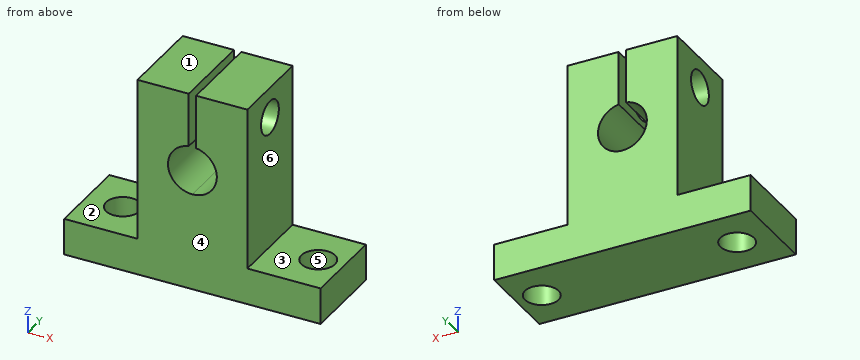
```python
from build123d import *

# Parameters (mm, degrees)
F1_DEPTH = 14
F2_R     = 2.75
F3_DEPTH = 6
F4_R     = 2.75
F5_DEPTH = 9
F6_R     = 2.75
F7_DEPTH = 9


with BuildPart() as f1:
    # F0 (on Front) → F1 (new body)
    with BuildSketch(Plane.XZ):
        with BuildLine():
            Line((-66.492734, 17.676073), (-45.492734, 17.676073))
            Line((-45.492734, 17.676073), (-24.492734, 17.676073))
            Line((-24.492734, 17.676073), (-24.492734, 23.676073))
            Line((-24.492734, 23.676073), (-36.492734, 23.676073))
            Line((-36.492734, 23.676073), (-36.492734, 50.476073))
            Line((-36.492734, 50.476073), (-44.892734, 50.476073))
            Line((-44.892734, 50.476073), (-44.892734, 41.630817))
            ThreePointArc((-44.892734, 41.630817), (-41.504064, 37.375221), (-45.492734, 33.676073))
            ThreePointArc((-45.492734, 33.676073), (-49.481404, 37.375221), (-46.092734, 41.630817))
            Line((-46.092734, 41.630817), (-46.092734, 50.476073))
            Line((-46.092734, 50.476073), (-54.492734, 50.476073))
            Line((-54.492734, 50.476073), (-54.492734, 23.676073))
            Line((-54.492734, 23.676073), (-66.492734, 23.676073))
            Line((-66.492734, 23.676073), (-66.492734, 17.676073))
        make_face()
    extrude(amount=F1_DEPTH)

    # F2 (on face) → F3 (cut)
    with BuildSketch(Plane.XY.offset(23.676073)):
        with Locations((-60.588689, -6.999696)):
            Circle(F2_R)
        with Locations((-28.588689, -6.999696)):
            Circle(F2_R)
    extrude(amount=-F3_DEPTH, mode=Mode.SUBTRACT)

    # F4 (on face) → F5 (cut)
    with BuildSketch(Plane.YZ.offset(-36.492734)):
        with Locations((-7, 45.476073)):
            Circle(F4_R)
    extrude(amount=-F5_DEPTH, mode=Mode.SUBTRACT)

    # F6 (on face) → F7 (cut)
    with BuildSketch(Plane(origin=(-54.492734, 0, 0), x_dir=(0, -1, 0), z_dir=(-1, 0, 0))):
        with Locations((7, 45.476073)):
            Circle(F6_R)
    extrude(amount=-F7_DEPTH, mode=Mode.SUBTRACT)


solid = f1.part
```
The listing builds one solid part. Answer for the finished solid, in the listing's coordinates (mm). Face numbers are marked on the shaded views. A direction names the side the tool comes from. Give positions to 0.01 mm unless a question says otherwise; leave off trailing zeros. Order: outer loops, then holes, each group sorted by start corner. A loop starts at its lowest first (then second) coordinate and runs counter-clockwise, first axis right, second up. Notation, with made-up numbers: (27.5, 66) - (74.5, 66) arc R24 cw to (74.5, 90) - close; hole circle Ø7 at (-9.75, -38.75). An arc over 180 degrees is marked (long way). Answer in a Markdown table with one row per item. Add a question column.
Q1. For a pull along Y with two mould halves and no side action, classify the marked faces 4, 5 and 6 as released by +Y, released by -Y, zero draft, split by the parting line, or undercut.
Q2. The part is cut by section D-D (y = -7.5). Determine the outline of the cut face in (x, z), then the cut area to 3 significant figures.
Q3. Find the intervals of material crossed by line 1 along X through (y, z) = (-13, 48); line 2 along X through (y, z) = (-9, 37.5); line 3 along Z through (x, y) = (-51.5, -7), in increasing order. Write a range as [from, to].
Q4. Given P1, Ø2.5, axis at y = -4.5, z = 46.5, coming from the -X side; P2, Ø6, axis at x = -31.5, y = -10.5, coming from the +Z side; P3, Ø1.5, axis at y = -6, z = 37.5, coming from the +X side, each flat-ended and moving along its own axis, determine where each tip first touches the part or whether it passes through.
Q5. The part is cut by section A-A (z = 36.5). Determine the outline of the cut face in (x, y).
Q6. The part is cut by section B-B (y = -2.5). Determine the outline of the cut face in (x, z), then the cut area to 3 significant figures.
Q7. Which of the six approach directions +Z, -Z, +X, -X, +Y, -Y give full straight-line access (tool end or side, diameter ignored) to the marked faces 1, 2 and 3?
Q8. The part is cut by section C-C (x = -59). Determine the outline of the cut face in (y, z).
Determined:
| question | item | result |
|---|---|---|
| 1 | face 4 | released by -Y |
| 1 | face 5 | undercut |
| 1 | face 6 | zero draft |
| 2 | outline | (-66.49, 17.68) - (-63.29, 17.68) - (-63.29, 23.68) - (-66.49, 23.68) - close; (-57.88, 17.68) - (-31.29, 17.68) - (-31.29, 23.68) - (-36.49, 23.68) - (-36.49, 42.77) - (-44.89, 42.77) - (-44.89, 41.63) arc R4 cw (long way) to (-46.09, 41.63) - (-46.09, 42.77) - (-54.49, 42.77) - (-54.49, 23.68) - (-57.88, 23.68) - close; (-54.49, 48.18) - (-46.09, 48.18) - (-46.09, 50.48) - (-54.49, 50.48) - close; (-44.89, 48.18) - (-36.49, 48.18) - (-36.49, 50.48) - (-44.89, 50.48) - close; (-25.88, 17.68) - (-24.49, 17.68) - (-24.49, 23.68) - (-25.88, 23.68) - close |
| 2 | area | 518 mm² |
| 3 | line 1 | x = [-54.49, -46.09], [-44.89, -36.49] |
| 3 | line 2 | x = [-54.49, -49.49], [-41.5, -36.49] |
| 3 | line 3 | z = [17.68, 42.73], [48.23, 50.48] |
| 4 | P1 | stops at x = -54.49 |
| 4 | P2 | stops at z = 23.68 |
| 4 | P3 | stops at x = -36.49 |
| 5 | outline | (-54.49, -14) - (-49.32, -14) - (-49.32, 0) - (-54.49, 0) - close; (-41.67, -14) - (-36.49, -14) - (-36.49, 0) - (-41.67, 0) - close |
| 6 | outline | (-66.49, 17.68) - (-24.49, 17.68) - (-24.49, 23.68) - (-36.49, 23.68) - (-36.49, 50.48) - (-44.89, 50.48) - (-44.89, 41.63) arc R4 cw (long way) to (-46.09, 41.63) - (-46.09, 50.48) - (-54.49, 50.48) - (-54.49, 23.68) - (-66.49, 23.68) - close |
| 6 | area | 674 mm² |
| 7 | face 1 | +Z, +X, -X, +Y, -Y |
| 7 | face 2 | +Z, -X, +Y, -Y |
| 7 | face 3 | +Z, +X, +Y, -Y |
| 8 | outline | (-14, 17.68) - (-9.24, 17.68) - (-9.24, 23.68) - (-14, 23.68) - close; (-4.76, 17.68) - (0, 17.68) - (0, 23.68) - (-4.76, 23.68) - close |
